Input: dimensioned drawing with shaded views. Units: mm. Origin: part minimum x, y, z. A direction names the side the tool comes from. Coordinates: 2 decimals unless noted, no trailing zeros. Order: outer loops, then holes, each group sorted by start corner. A loop starts at its lowest first (then second) coordinate and runs counter-clockwise, first axis right, second up. Notation, with made-up numbers: (84, 15.5) -> (126, 15.5) arc R22 ccw to (126, 42.5) -> close; hole circle Ø2 at (27, 16). An arc over 180 degrees is marked (long way). Put each result on its own line as item: value.
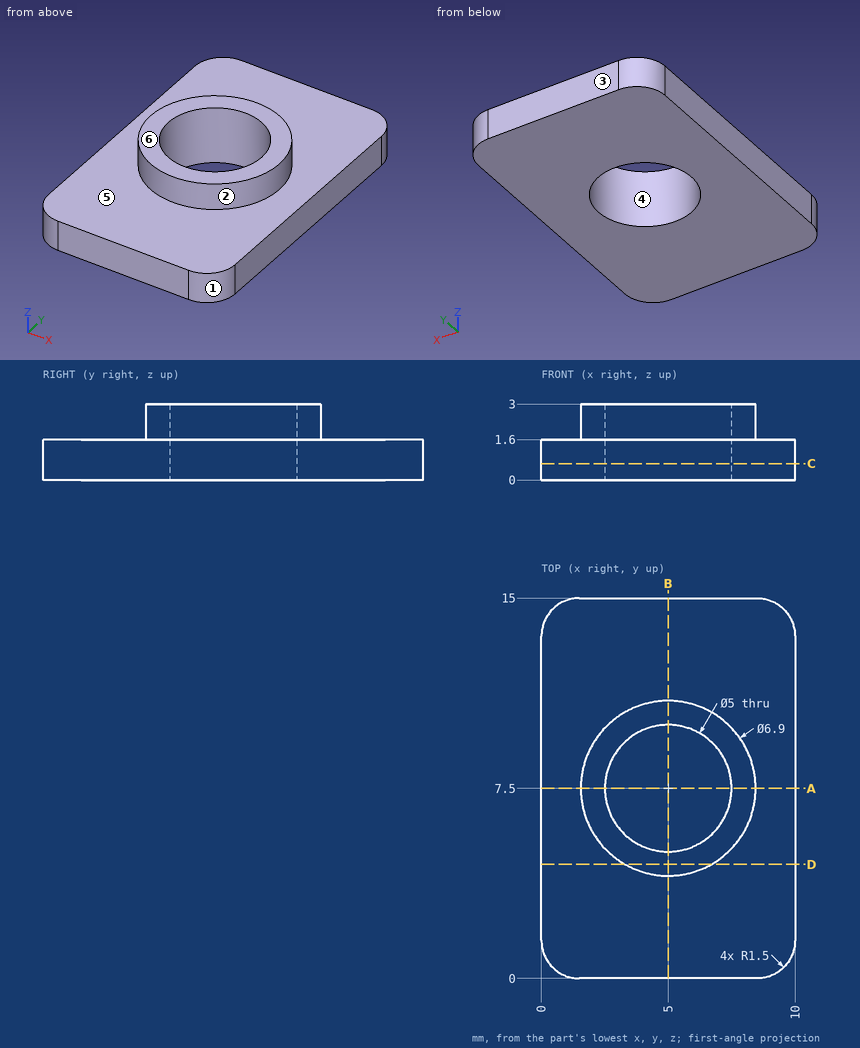
1. Cut plane B-B on x = 5. Output: boundary loops of the cut face in (y, z), plus the area to 3 significant figures.
Numbers:
outline: (0, 0) -> (5, 0) -> (5, 3) -> (4.05, 3) -> (4.05, 1.6) -> (0, 1.6) -> close; (10, 0) -> (15, 0) -> (15, 1.6) -> (10.95, 1.6) -> (10.95, 3) -> (10, 3) -> close
area: 18.7 mm2
2. First-contact query: pin 1 (2 mm diameter, centred on x = 2.5, y = 10, fed in from +Z). Flat tip, straight axial feed; report the tip coordinate or a pass-through.
Numbers:
pin 1: stops at z = 3
3. Ray query, line 1 along Y through (x, z) = (5, 1.75); line 2 along Z through (x, y) = (0.5, 7.5); line 3 along X through (y, z) = (7, 2.2). Return the intervals inside material, ascending.
Numbers:
line 1: y = 4.05 to 5, 10 to 10.95
line 2: z = 0 to 1.6
line 3: x = 1.59 to 2.55, 7.45 to 8.41
4. Pull-direction query (Y, two-part tool) for the marked faces 1, 2, 3 and 4; classes: pulls with the +Y half, pulls with the -Y half, needs draft (parallel to the pull), parting line crosses it, or undercut.
Numbers:
face 1: pulls with the -Y half
face 2: parting line crosses it
face 3: pulls with the +Y half
face 4: undercut
5. Cut plane D-D on y = 4.5. Output: boundary loops of the cut face in (x, z).
Numbers:
outline: (0, 0) -> (10, 0) -> (10, 1.6) -> (6.7, 1.6) -> (6.7, 3) -> (3.3, 3) -> (3.3, 1.6) -> (0, 1.6) -> close
6. Set-up query: the marked faces 5 and 6. Return all of +Z, -Z, +X, -X, +Y, -Y with unobstructed straight access to the full face (end or side cutting, diameter ignored); none if empty.
Numbers:
face 5: +Z
face 6: +Z, +X, -X, +Y, -Y
7. Cut plane A-A on y = 7.5. Output: boundary loops of the cut face in (x, z), plus the area to 3 significant figures.
Numbers:
outline: (0, 0) -> (2.5, 0) -> (2.5, 3) -> (1.55, 3) -> (1.55, 1.6) -> (0, 1.6) -> close; (7.5, 0) -> (10, 0) -> (10, 1.6) -> (8.45, 1.6) -> (8.45, 3) -> (7.5, 3) -> close
area: 10.7 mm2
8. Cut plane C-C on z = 0.65. Output: boundary loops of the cut face in (x, y).
Numbers:
outline: (0, 1.5) arc R1.5 ccw to (1.5, 0) -> (8.5, 0) arc R1.5 ccw to (10, 1.5) -> (10, 13.5) arc R1.5 ccw to (8.5, 15) -> (1.5, 15) arc R1.5 ccw to (0, 13.5) -> close; hole circle Ø5 at (5, 7.5)
